Input: part model. Units: mm. Frame: model coordinates. A direction names the side the tool comes from. Round coordinates to 2 decimals unless told otherwise and drop trailing zeros. Loops run counter-clockwise (first coordinate to the right, second up) from the corner with the lowest first, then second, coordinate; pieces in that order, holes last.
(1) Cut plane C-C, the plane y = 22. Output: boundary loops of the cut face in (x, z).
(2) First-contact query: pin 1 Ø1.5 at (x, y) = (-30, 17) entering from -Z. Flat tip, straight axial feed; report the tip coordinate or a pass-through.
(3) Cut plane B-B, the plane x = -17. Output: boundary loops of the cut face in (y, z).
(4) Line query: line 1 (Y direction, x = 0, z = -4.75); line 2 (Y direction, x = 0, z = -1.5); line 3 (X direction, y = 28, z = -4.5) (3 decimals). Output: solid intervals per line, ascending.
(5) Cut plane A-A, the plane z = -4.25. Give the number of separate pieces and of enclosed holes in the cut face, and give its area (3 significant figures).
(6) Draft query along Y for faces 1 (the face through (40, -1, 0)), 2 (the face through (20.744, 0.245, -1.141)), 3 (the face through (-31.96, -31.68, 0.11)). Return one class per face: released by +Y, released by -Y, zero draft, split by the parting line, or undercut.
(7) Access query for faces 4 (the face through (20.02, -5.93, 11.51)), 5 (the face through (-19.531, 1.421, -0.465)), 6 (the face through (4.071, -19.953, -10.206)), 7 (the face through (-34, -34, 8)). Directions: +Z, -Z, +X, -X, +Y, -Y. A direction counts if a zero-diameter tool reaches every point of the face in a straight line with its end or side. Return the directions, or none.
(8) Cut plane D-D, the plane x = -26. Output: boundary loops of the cut face in (y, z).
from build123d import *

# Parameters (mm, degrees)
SKETCH1_W                = 80
SKETCH1_H                = 80
SKETCH1_R                = 37.5
BOSS_EXTRUDE1_DEPTH      = 12.5
BOSS_EXTRUDE1_DEPTH_BACK = 12.5
SKETCH2_R                = 60
SKETCH2_R_2              = 45
CUT_EXTRUDE1_DEPTH       = 8
CUT_EXTRUDE1_DEPTH_BACK  = 8
SKETCH3_R                = 2
CUT_EXTRUDE2_DEPTH       = 26
SKETCH4_R                = 10
BOSS_EXTRUDE2_DEPTH      = 2
SKETCH5_R                = 7.5
BOSS_EXTRUDE3_DEPTH      = 23
BOSS_EXTRUDE9_START      = -17.942054
BOSS_EXTRUDE9_DEPTH      = 35.442054
CIRPATTERN1_COUNT        = 6


with BuildPart() as part:
    # Sketch1 → Boss-Extrude1 (new body, two sides)
    with BuildSketch(Plane.XY) as boss_extrude1_sk:
        Rectangle(SKETCH1_W, SKETCH1_H)
        Circle(SKETCH1_R, mode=Mode.SUBTRACT)
    extrude(amount=BOSS_EXTRUDE1_DEPTH)
    extrude(boss_extrude1_sk.sketch, amount=-BOSS_EXTRUDE1_DEPTH_BACK)

    # Sketch2 → Cut-Extrude1 (cut, two sides)
    with BuildSketch(Plane.XY) as cut_extrude1_sk:
        Circle(SKETCH2_R)
        Circle(SKETCH2_R_2, mode=Mode.SUBTRACT)
    extrude(amount=CUT_EXTRUDE1_DEPTH, mode=Mode.SUBTRACT)
    extrude(cut_extrude1_sk.sketch, amount=-CUT_EXTRUDE1_DEPTH_BACK, mode=Mode.SUBTRACT)

    # Sketch3 → Cut-Extrude2 (cut, through all)
    with BuildSketch(Plane.XY.offset(12.5)):
        with Locations((-36, 36)):
            Circle(SKETCH3_R)
        with Locations((36, 36)):
            Circle(SKETCH3_R)
        with Locations((36, -36)):
            Circle(SKETCH3_R)
        with Locations((-36, -36)):
            Circle(SKETCH3_R)
    extrude(amount=-CUT_EXTRUDE2_DEPTH, mode=Mode.SUBTRACT)

    # Sketch4 → Boss-Extrude2 (add)
    with BuildSketch(Plane.XY.offset(12.5)):
        with BuildLine():
            Line((18.549623759, 32.590818621), (-7.057093407, 7.085014654))
            ThreePointArc((-7.057093407, 7.085014654), (-4.306304625, 9.025283401), (-1.067547722, 9.942853809))
            Line((-1.067547722, 9.942853809), (20.484975285, 31.410440741))
            ThreePointArc((20.484975285, 31.410440741), (19.526220925, 32.015257244), (18.549623759, 32.590818621))
        make_face()
        Circle(SKETCH4_R)
        with BuildLine():
            ThreePointArc((-7.085014654, -7.057093407), (-9.025283401, -4.306304625), (-9.942853809, -1.067547722))
            Line((-9.942853809, -1.067547722), (-31.410440741, 20.484975285))
            ThreePointArc((-31.410440741, 20.484975285), (-32.015257244, 19.526220925), (-32.590818621, 18.549623759))
            Line((-32.590818621, 18.549623759), (-7.085014654, -7.057093407))
        make_face()
        with BuildLine():
            Line((32.590818621, -18.549623759), (7.085014654, 7.057093407))
            ThreePointArc((7.085014654, 7.057093407), (9.025283401, 4.306304625), (9.942853809, 1.067547722))
            Line((9.942853809, 1.067547722), (31.410440741, -20.484975285))
            ThreePointArc((31.410440741, -20.484975285), (32.015257244, -19.526220925), (32.590818621, -18.549623759))
        make_face()
        with BuildLine():
            ThreePointArc((7.057093407, -7.085014654), (4.306304625, -9.025283401), (1.067547722, -9.942853809))
            Line((1.067547722, -9.942853809), (-20.484975285, -31.410440741))
            ThreePointArc((-20.484975285, -31.410440741), (-19.526220925, -32.015257244), (-18.549623759, -32.590818621))
            Line((-18.549623759, -32.590818621), (7.057093407, -7.085014654))
        make_face()
    extrude(amount=-BOSS_EXTRUDE2_DEPTH)

    # Sketch5 → Boss-Extrude3 (add)
    with BuildSketch(Plane(origin=(0, 0, 10.5), x_dir=(-1, 0, 0), z_dir=(0, 0, -1))):
        Circle(SKETCH5_R)
    extrude(amount=BOSS_EXTRUDE3_DEPTH)

    # Sketch7 → Boss-Extrude9 (add)
    with BuildSketch(Plane(origin=(20, 0, 0), x_dir=(0, 0, -1), z_dir=(1, 0, 0)).offset(BOSS_EXTRUDE9_START)):
        Polygon((9.730274214, -7.212132837), (-9.063025071, 4.533679216), (-8.124052437, 6.03603543), (10.669246848, -5.709776623), align=None)
    boss_extrude9 = extrude(amount=BOSS_EXTRUDE9_DEPTH)

    # CirPattern1: Boss-Extrude9 ×6 about axis
    cirpattern1_axis = Axis((0, 0, 0), (0, 0, 1))
    for i in range(1, CIRPATTERN1_COUNT):
        add(boss_extrude9.rotate(cirpattern1_axis, i * 360 / CIRPATTERN1_COUNT))


solid = part.part
Reported:
1. outline: (-40, -12.5) - (-30.37, -12.5) - (-30.37, 12.5) - (-40, 12.5) - (-40, 8) - (-39.26, 8) - (-39.26, -8) - (-40, -8) - close; (-19.67, 8.12) - (-6.11, -10.67) - (-4.37, -9.73) - (-17.94, 9.06) - close; (5.73, 8.12) - (19.29, -10.67) - (21.03, -9.73) - (7.47, 9.06) - close; (7.92, 10.5) - (11.04, 10.5) - (11.04, 12.5) - (7.92, 12.5) - close; (30.37, -12.5) - (40, -12.5) - (40, -8) - (39.26, -8) - (39.26, 8) - (40, 8) - (40, 12.5) - (30.37, 12.5) - close
2. pin 1: stops at z = 10.5
3. outline: (-40, -12.5) - (-33.43, -12.5) - (-33.43, 1.65) - (-18.03, -10.67) - (-15.02, -9.73) - (-33.43, 4.99) - (-33.43, 12.5) - (-40, 12.5) - close; (-31.05, 10.5) - (-27.94, 10.5) - (-27.94, 12.5) - (-31.05, 12.5) - close; (-6.04, 8.12) - (5.71, -10.67) - (7.21, -9.73) - (-4.53, 9.06) - close; (2.9, 10.5) - (6.02, 10.5) - (6.02, 12.5) - (2.9, 12.5) - close; (17.37, 8.12) - (33.43, -4.72) - (33.43, -12.5) - (40, -12.5) - (40, 12.5) - (33.43, 12.5) - (33.43, -1.38) - (20.38, 9.06) - close
4. line 1: y = -40 to -37.5, -8.2 to 8.2, 37.5 to 40
4. line 2: y = -40 to -37.5, -7.5 to 7.5, 37.5 to 40
4. line 3: x = -35.228 to -24.945, -14.025 to -11.613, 18.307 to 20.719, 24.945 to 35.228
5. separate pieces: 1
5. enclosed holes: 6
5. area: 1,950 mm2
6. face 1: zero draft
6. face 2: undercut
6. face 3: released by -Y
7. face 4: +Z
7. face 5: none
7. face 6: -Z
7. face 7: -X, -Y
8. outline: (-40, -12.5) - (-27.02, -12.5) - (-27.02, 12.5) - (-40, 12.5) - (-40, 8) - (-36.73, 8) - (-36.73, -8) - (-40, -8) - close; (-6.04, 8.12) - (5.71, -10.67) - (7.21, -9.73) - (-4.53, 9.06) - close; (11.93, 10.5) - (15.05, 10.5) - (15.05, 12.5) - (11.93, 12.5) - close; (27.02, -12.5) - (40, -12.5) - (40, -8) - (36.73, -8) - (36.73, 8) - (40, 8) - (40, 12.5) - (27.02, 12.5) - close
